For this review, use the dimensioned drawing (mm, ordinates from the lowest corner) and the shaded views. Give positions to 0.01 mm unless a question says otherwise; leave off trailing zeros. Loops run counter-clockwise (first coordinate to the right, second up) from the corner with the lowest first, then second, coordinate; pieces in that order, holes last. Notation, with made-up numbers: M 42,75 L 74,75 A21 cw 74,83 Z; hole C -34,75.25 d5. An arc over 180 degrees is marked long. Use a Markdown table: item, result. Add a question column.
(1) For probe 1 along X at (y, z) = (10, 3); probe 2 along Z at (x, y) = (1.15, 6) (1 decimal); probe 3 along X at (y, z) = (2.5, 3.5), list the stretches that pass through material, from the lowest coordinate up.
(2) Add section A-A, the plane y = 2. Give the boundary of the cut face in (x, z).
(3) Add section C-C, the plane x = 4.3. Give the boundary of the cut face in (y, z) (1 decimal).
(4) Add section B-B, the plane z = 0.35. Give the boundary of the cut face in (x, y).
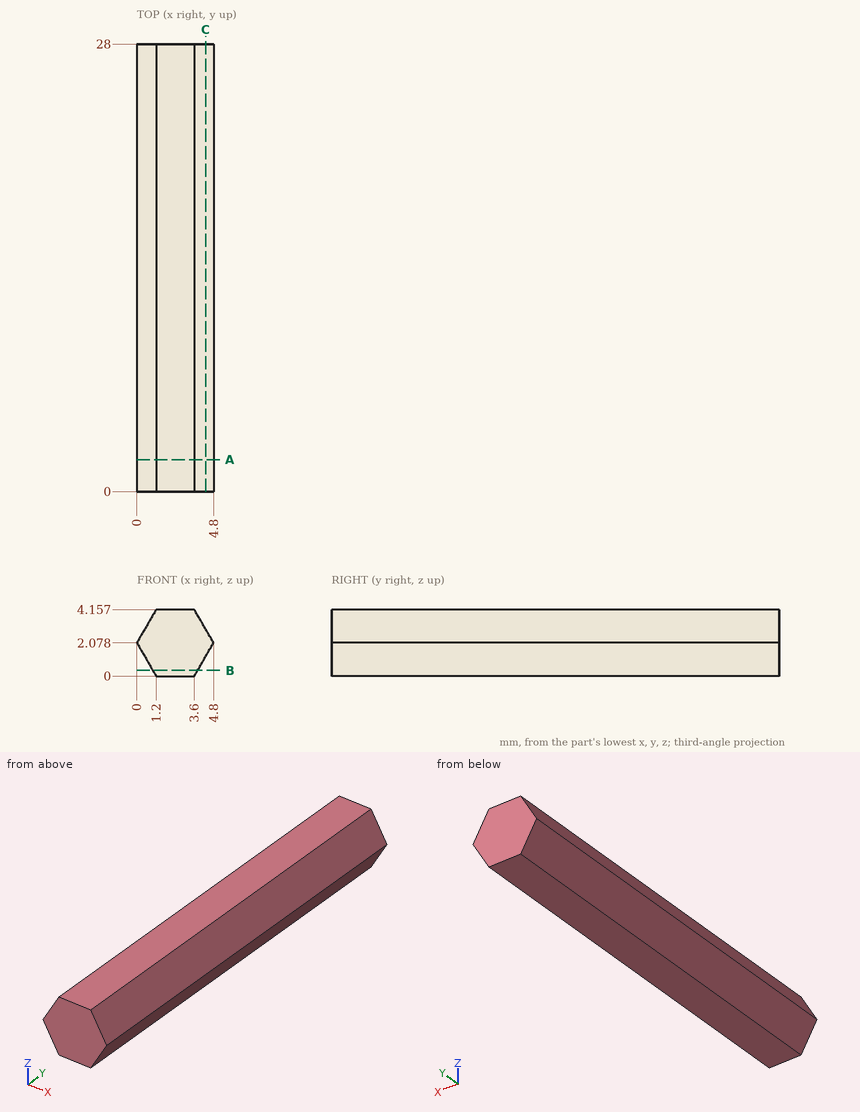
Established:
| question | item | result |
|---|---|---|
| 1 | probe 1 | 0.53 to 4.27 |
| 1 | probe 2 | 0.1 to 4.1 |
| 1 | probe 3 | 0.82 to 3.98 |
| 2 | outline | M 0,2.08 L 1.2,0 L 3.6,0 L 4.8,2.08 L 3.6,4.16 L 1.2,4.16 Z |
| 3 | outline | M 0,1.2 L 28,1.2 L 28,2.9 L 0,2.9 Z |
| 4 | outline | M 1,0 L 3.8,0 L 3.8,28 L 1,28 Z |
